from build123d import *

# Parameters (mm, degrees)
BOSS_EXTRUDE1_DEPTH      = 5
BOSS_EXTRUDE1_DEPTH_BACK = 5
SKETCH2_R                = 1.55
CUT_EXTRUDE1_START       = -10
CUT_EXTRUDE1_DEPTH       = 10
FILLET1_R                = 1


with BuildPart() as part:
    # Sketch2 → Boss-Extrude1 (new, two sides: drawn at the far end of the back side and taken through both)
    with BuildSketch(Plane.XY.offset(-BOSS_EXTRUDE1_DEPTH_BACK)):
        with BuildLine():
            Line((2.905523423, 2.749169627), (-11.641714865, 18.12375444))
            ThreePointArc((-11.641714865, 18.12375444), (-18.21926668, 19.574482524), (-22, 14))
            ThreePointArc((-22, 14), (-42.474078457, 23.622085), (-60.163399658, 37.723869421))
            ThreePointArc((-60.163399658, 37.723869421), (-76.495910352, 60.486816081), (-80.043672644, 88.277390543))
            ThreePointArc((-80.043672644, 88.277390543), (-85.99568578, 94.999998449), (-91.957360362, 88.285956923))
            ThreePointArc((-91.957360362, 88.285956923), (-84.145355247, 58.049091263), (-68.630234445, 30.946019566))
            ThreePointArc((-68.630234445, 30.946019566), (-38.101001964, 6.292742427), (-0.232587209, -3.993232173))
            ThreePointArc((-0.232587209, -3.993232173), (3.626450401, -1.687855885), (2.905523423, 2.749169627))
        make_face()
        with Locations((-86, 89)):
            Circle(SKETCH2_R, mode=Mode.SUBTRACT)
        with Locations((-16, 14)):
            Circle(SKETCH2_R, mode=Mode.SUBTRACT)
        with Locations((-3.6022, 2.7054)):
            Circle(SKETCH2_R, mode=Mode.SUBTRACT)
    extrude(amount=BOSS_EXTRUDE1_DEPTH + BOSS_EXTRUDE1_DEPTH_BACK)

    # Sketch3 → Cut-Extrude1 (cut)
    with BuildSketch(Plane.XY.offset(5).offset(CUT_EXTRUDE1_START)):
        with BuildLine():
            Line((-19.012966708, -1.001561409), (-19.012966708, 9.18151319))
            ThreePointArc((-19.012966708, 9.18151319), (-15.891446961, 8.318098931), (-12.805184231, 9.300113222))
            Line((-12.805184231, 9.300113222), (-12.805184231, -2.418437298))
            ThreePointArc((-12.805184231, -2.418437298), (-15.920894449, -1.76178205), (-19.012966708, -1.001561409))
        make_face()
    extrude(amount=CUT_EXTRUDE1_DEPTH, mode=Mode.SUBTRACT)

    # Fillet1
    fillet1_edges = [part.edges().sort_by_distance(p)[0] for p in [
        (-12.805184231, -2.418437298, 0),
        (-19.012966708, -1.001561409, 0),
        (-19.012966708, 9.18151319, 0),
        (-12.805184231, 9.300113222, 0),
    ]]
    fillet(fillet1_edges, radius=FILLET1_R)


solid = part.part
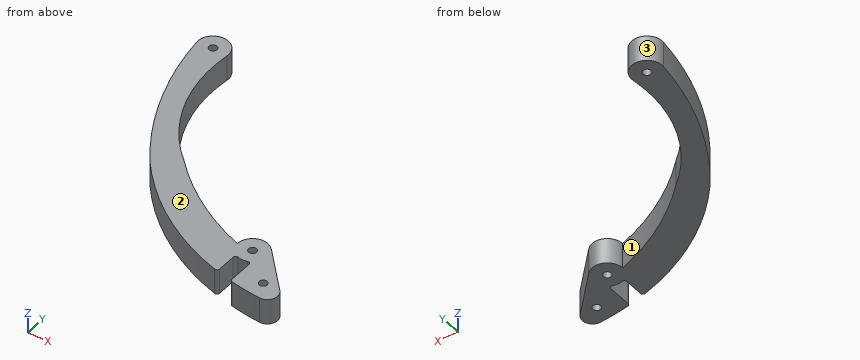
Work out the finished part from the listing and answer in its coordinate system (mm). Face numbers are marked on the shaded views. Coordinates: 2 decimals unless noted, no trailing zeros. Write each loop counter-clockwise with the first axis right and the second up, starting at its lowest first coordinate (ties: lowest second). Pieces come first, ordered by that corner, then holes.
1. The part is cut by section D-D, the plane y = 80. Write down the section's boundary in (x, z).
Results list:
outline: (-90.66, -5) - (-80.44, -5) - (-80.44, 5) - (-90.66, 5) - close
2. For a pull along X with two mould halves and no side action, classify the marked faces 1, 2 and 3 as +X half, -X half, draft (parallel to the pull), parting line (faces both ways), or undercut.
Results list:
face 1: undercut
face 2: draft
face 3: parting line
3. Flat-ended cylindrical pins translate along their axes: pin 1 (1.5 mm diameter, centred on x = -15, z = 1.5, fed in from +Y); pin 2 (4 mm diameter, centred on x = -37.5, z = -3.5, fed in from -Y); pin 3 (4 mm diameter, centred on x = -46.5, z = 2.5, fed in from -Y). Find the tip coordinate at first contact, or state that the pin passes through.
Results list:
pin 1: stops at y = 19.99
pin 2: stops at y = 5.01
pin 3: stops at y = 9.88
4. The part is cut by section A-A, the plane x = -16. Write down the section's boundary in (y, z), and give its area (3 significant figures).
Results list:
outline: (8.32, -5) - (12.45, -5) - (12.45, 5) - (8.32, 5) - close; (15.55, -5) - (20, -5) - (20, 5) - (15.55, 5) - close
area: 85.8 mm2
5. The part is cut by section C-C, the plane x = -86. Write down the section's boundary in (y, z).
Results list:
outline: (62.91, -5) - (87.45, -5) - (87.45, 5) - (62.91, 5) - close; (90.55, -5) - (95, -5) - (95, 5) - (90.55, 5) - close
6. Consider line 1 along X through (y, z) = (89, -1.5); line 2 along X through (y, z) = (19, -1.75); line 3 along X through (y, z) = (62.5, -3.5). Determine where each line is inside the solid, lowest interval first.
Results list:
line 1: x = -92 to -87.55, -84.45 to -80
line 2: x = -57 to -34.15, -19.32 to -12.68
line 3: x = -85.85 to -77.24
7. The part is cut by section B-B, the plane z = 2. Write down the section's boundary in (x, y), and give its area (3 significant figures).
Results list:
outline: (-91.96, 88.29) arc R117.28 ccw to (-68.63, 30.95) arc R95.44 ccw to (-20.28, -0.66) arc R1 ccw to (-19.01, 0.31) - (-19.01, 7.63) arc R1 cw to (-17.71, 8.58) arc R5.68 ccw to (-14.13, 8.63) arc R1 cw to (-12.81, 7.69) - (-12.81, -1.59) arc R1 ccw to (-11.99, -2.57) arc R95.44 ccw to (-0.23, -3.99) arc R4 ccw to (2.91, 2.75) - (-11.64, 18.12) arc R6 ccw to (-22, 14) arc R97.02 cw to (-60.16, 37.72) arc R57.13 cw to (-80.04, 88.28) arc R6 ccw (long way) to start; hole circle Ø3.1 at (-86, 89); hole circle Ø3.1 at (-16, 14); hole circle Ø3.1 at (-3.6, 2.71)
area: 1,580 mm2
